```python
from build123d import *

# Parameters (mm, degrees)
SKETCH1_W                      = 121.5
SKETCH1_H                      = 36.5
SKETCH1_W_2                    = 115.5
SKETCH1_H_2                    = 30.5
BOSS_EXTRUDE1_DEPTH            = 3
SKETCH1_3_W                    = 121.5
SKETCH1_3_H                    = 36.5
SKETCH1_3_W_2                  = 115.5
SKETCH1_3_H_2                  = 30.5
BOSS_EXTRUDE2_DEPTH            = 17
BOSS_EXTRUDE3_DEPTH            = 118.5
BOSS_EXTRUDE3_DEPTH_BACK       = 3
CBORE_FOR_M5_SHCS1_D           = 5.3
CBORE_FOR_M5_SHCS1_CBORE_D     = 10
CBORE_FOR_M5_SHCS1_CBORE_DEPTH = 13
FILLET1_R                      = 2


with BuildPart() as part:
    # Sketch1 → Boss-Extrude1 (new body)
    # profile 1 of 2: a face of its own
    with BuildSketch(Plane.XY):
        with Locations((57.75, 15.25)):
            Rectangle(SKETCH1_W, SKETCH1_H)
        with Locations((57.75, 15.25)):
            Rectangle(SKETCH1_W_2, SKETCH1_H_2, mode=Mode.SUBTRACT)
    # profile 2 of 2: a face of its own
    with BuildSketch(Plane.XY):
        with Locations((57.75, 15.25)):
            Rectangle(SKETCH1_W_2, SKETCH1_H_2)
    extrude(amount=-BOSS_EXTRUDE1_DEPTH)

    # Sketch1<3> → Boss-Extrude2 (add)
    with BuildSketch(Plane.XY):
        with Locations((57.75, 15.25)):
            Rectangle(SKETCH1_3_W, SKETCH1_3_H)
        with Locations((57.75, 15.25)):
            Rectangle(SKETCH1_3_W_2, SKETCH1_3_H_2, mode=Mode.SUBTRACT)
    extrude(amount=BOSS_EXTRUDE2_DEPTH)

    # Sketch2 → Boss-Extrude3 (add, two sides: drawn at the far end of the back side and taken through both)
    with BuildSketch(Plane(origin=(0, 0, 0), x_dir=(0, 0, -1), z_dir=(1, 0, 0)).offset(-BOSS_EXTRUDE3_DEPTH_BACK)):
        with BuildLine():
            Line((3, 33.5), (3, 12))
            Line((3, 12), (23, 12))
            Line((23, 12), (23, 15))
            ThreePointArc((23, 15), (22.822381628, 15.823969176), (22.321074797, 16.501586289))
            Line((22.321074797, 16.501586289), (3, 33.5))
        make_face()
    extrude(amount=BOSS_EXTRUDE3_DEPTH + BOSS_EXTRUDE3_DEPTH_BACK)

    # CBORE for M5 SHCS1 (through all)
    with Locations(Plane(origin=(0, 33.5, 0), x_dir=(1, 0, 0), z_dir=(0, 1, 0))):
        with Locations((7.75, 13), (41.083333333, 13), (74.416666667, 13), (107.75, 13)):
            CounterBoreHole(CBORE_FOR_M5_SHCS1_D / 2, CBORE_FOR_M5_SHCS1_CBORE_D / 2, CBORE_FOR_M5_SHCS1_CBORE_DEPTH)

    # Fillet1
    fillet1_edges = [part.edges().sort_by_distance(p)[0] for p in [
        (57.75, 33.5, -3),
        (57.75, 0, 0),
        (115.5, 0, 8.5),
        (0, 0, 8.5),
        (-3, 13.5, -23),
        (-3, 15.823969176, -22.822381628),
        (-3, 25.000793144, -12.660537398),
        (57.75, 12, -3),
        (118.5, 13.5, -23),
        (118.5, 15.823969176, -22.822381628),
        (118.5, 25.000793144, -12.660537398),
        (118.5, -3, 7),
        (-3, -3, 7),
        (-3, 33.5, 7),
        (118.5, 33.5, 7),
    ]]
    fillet(fillet1_edges, radius=FILLET1_R)


solid = part.part
```
Could you check a few things on this model? Use its own coordinates, in mm. A direction names the side the tool comes from. Round coordinates to 2 decimals unless told otherwise and drop trailing zeros. Loops run counter-clockwise (first coordinate to the right, second up) from the corner with the lowest first, then second, coordinate; pieces in that order, holes last.
Q1. I want a section at B-B (y = 8). Write out the boundary of the cut face in (x, z).
Q2. On a 3-axis mill with a long thin cutter (end or side, diameter ignored), from which of +Z, -Z, +X, -X, +Y, -Y can I reach the whole of each face in a straight line? I mean faces 1 (the flat face through (57, 4, -3)), 2 (the cylindrical face through (-2.399, 24.439, -12.436)), 3 (the cylindrical face through (43.19, 16.19, -11.39)), 4 (the cylindrical face through (0.57, 0.6, 8.62)), 5 (the cylindrical face through (41, 24, -8)). Say none if no direction works.
Q3. For P1, Ø13, axis at x = 74.42, z = -13, coming from the -Y side; P2, Ø12, axis at x = 21.5, z = -14.5, coming from the +Y side; P3, Ø9, axis at x = 107.75, z = -13, coming from the +Y side; P4, Ø3, axis at x = 74.42, z = -13, coming from the -Y side, each with a flat end and sliding along its axis, tell me the tip position at first contact or that it passes through.
Q4. I want a section at D-D (x = 81). Write out the boundary of the cut face in (y, z), and give its area (3 significant figures).
Q5. Thinking about a two-plate mould opening in X: for faces 6 (the cylindrical face through (74.218, 23.967, -8.004)), 7 (the cylindrical face through (117.9, 32.93, 7.24)), 8 (the flat face through (-3, 15, 2)), 9 (the flat face through (77, 20.5, -15)), which applies, pulls with the +X half, pulls with the -X half, needs draft (parallel to the pull), parting line crosses it, or undercut?
Q6. Please list where these lines run through material, in increasing order: L1, parallel to X at y = 18, z = -13; L2, parallel to Y at x = 90.5, z = 9; L3, parallel to X at y = 22, z = 1.
Q7. I want a section at A-A (x = 7.75). Write out the boundary of the cut face in (y, z).
Q8. I want a section at C-C (z = 14). Write out the boundary of the cut face in (x, y).
Answer below:
1. outline: (-3, -3) - (118.5, -3) - (118.5, 17) - (115.5, 17) - (115.5, 0) - (0, 0) - (0, 17) - (-3, 17) - close
2. face 1: -Z, +X, -X, -Y
2. face 2: -Z, -X, +Y
2. face 3: +Y, -Y
2. face 4: +Z
2. face 5: +Y
3. P1: stops at y = 12
3. P2: stops at y = 28.66
3. P3: stops at y = 20.5
3. P4: passes through
4. outline: (-3, -3) - (10, -3) arc R2 cw to (12, -5) - (12, -23) - (15, -23) arc R2 ccw to (16.5, -22.32) - (33, -3.57) arc R2 ccw to (33.5, -2.25) - (33.5, 17) - (30.5, 17) - (30.5, 0) - (2, 0) arc R2 cw to (0, 2) - (0, 17) - (-3, 17) - close
4. area: 467 mm2
5. face 6: undercut
5. face 7: pulls with the +X half
5. face 8: pulls with the -X half
5. face 9: undercut
6. L1: x = -3 to 5.1, 10.4 to 38.43, 43.73 to 71.77, 77.07 to 105.1, 110.4 to 118.5
6. L2: y = -3 to 0, 30.5 to 33.5
6. L3: x = -3 to 0, 115.5 to 118.5
7. outline: (-3, -3) - (10, -3) arc R2 cw to (12, -5) - (12, -10.35) - (20.5, -10.35) - (20.5, -8) - (29.1, -8) - (33, -3.57) arc R2 ccw to (33.5, -2.25) - (33.5, 17) - (30.5, 17) - (30.5, 0) - (2, 0) arc R2 cw to (0, 2) - (0, 17) - (-3, 17) - close; (12, -23) - (15, -23) arc R2 ccw to (16.5, -22.32) - (20.5, -17.78) - (20.5, -15.65) - (12, -15.65) - close
8. outline: (-3, -1) arc R2 ccw to (-1, -3) - (116.5, -3) arc R2 ccw to (118.5, -1) - (118.5, 31.5) arc R2 ccw to (116.5, 33.5) - (-1, 33.5) arc R2 ccw to (-3, 31.5) - close; hole (0, 2) arc R2 ccw to (2, 0) - (113.5, 0) arc R2 ccw to (115.5, 2) - (115.5, 30.5) - (0, 30.5) - close
